Geometry check sheet. Reference: drawing and pictorial views, mm from the part's lowest x, y, z. Coordinates: 2 decimals unless noted, no trailing zeros. Write each loop counter-clockwise with the first axis right and the second up, starting at its lowest first coordinate (ties: lowest second). Pieces come first, ordered by that corner, then holes. Notation, with made-up numbers: (25, -13.75) -> (48, -13.75) arc R28 ccw to (48, 14.25) -> close; hole circle Ø3 at (38.5, -18.5). An arc over 180 degrees is marked (long way). Answer in a Markdown table with one row per item.
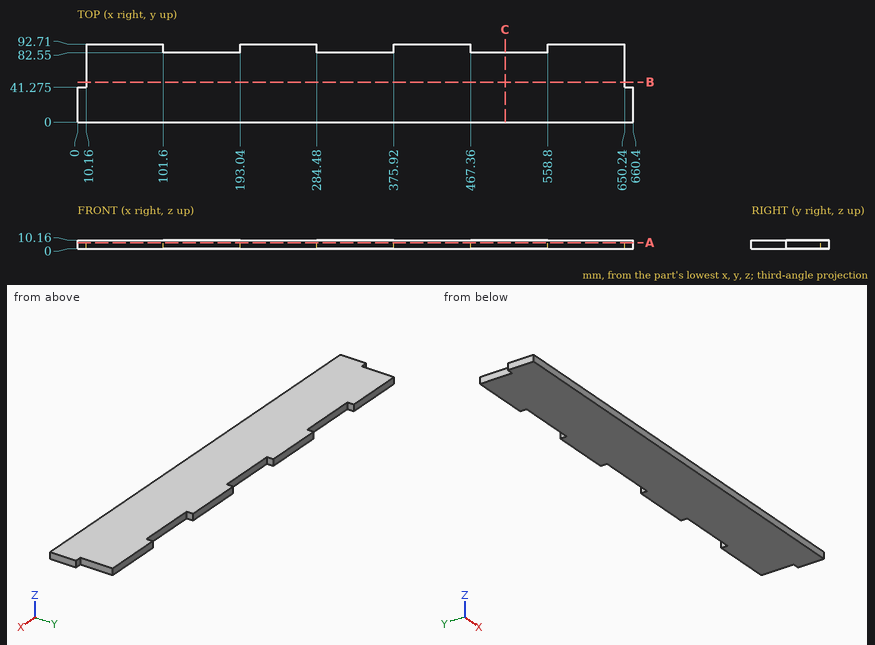
1. Section check C-C, the plane x = 508. Record the boundary of the cut face in (y, z).
Geometry says:
| item | result |
|---|---|
| outline | (0, 0) -> (82.55, 0) -> (82.55, 10.16) -> (0, 10.16) -> close |
2. Section check B-B, the plane y = 47.5. Record the boundary of the cut face in (x, z), plus the area to 3 significant figures.
Geometry says:
| item | result |
|---|---|
| outline | (10.16, 0) -> (650.24, 0) -> (650.24, 10.16) -> (10.16, 10.16) -> close |
| area | 6,500 mm^2 |
3. Depth check by flat-ended pin: P1, Ø6, axis at y = 49.5, z = 7.5, coming from the +X side; P2, Ø3, axis at x = 655.5, z = 2.5, coming from the +Y side (3 decimals); P3, Ø3, axis at x = 531, z = 3.5, coming from the +Y side. Enter the tip coordinate at first touch or a pass-through.
Geometry says:
| item | result |
|---|---|
| P1 | x = 650.24 |
| P2 | y = 41.275 |
| P3 | y = 82.55 |
4. Section check A-A, the plane z = 7. Record the boundary of the cut face in (x, y) (3 decimals).
Geometry says:
| item | result |
|---|---|
| outline | (0, 0) -> (660.4, 0) -> (660.4, 41.275) -> (650.24, 41.275) -> (650.24, 92.71) -> (558.8, 92.71) -> (558.8, 82.55) -> (467.36, 82.55) -> (467.36, 92.71) -> (375.92, 92.71) -> (375.92, 82.55) -> (284.48, 82.55) -> (284.48, 92.71) -> (193.04, 92.71) -> (193.04, 82.55) -> (101.6, 82.55) -> (101.6, 92.71) -> (10.16, 92.71) -> (10.16, 41.275) -> (0, 41.275) -> close |
5. Thickness scan on line 1 (X direction, y = 65, z = 3); line 2 (Y direction, x = 487.5, z = 9.5). Record the ranges inside material, lowest first. Write a range as from..to.
Geometry says:
| item | result |
|---|---|
| line 1 | 10.16..650.24 |
| line 2 | 0..82.55 |
